Build history of the part. All positions in model axes, mm. A direction names the side the tool comes from. Round coordinates to 2 decimals unless told otherwise and drop trailing zeros. Write each loop counter-clockwise with the first axis right and the second up, starting at its lowest first coordinate (ties: lowest second). Pieces come first, ordered by that corner, then holes.
Autodesk Inventor part; units mm, degrees
ref_plane "YZ Plane" through (0, 0, 0) normal (1, 0, 0) x (0, 1, 0)
ref_plane "XZ Plane" through (0, 0, 0) normal (0, 1, 0) x (-1, 0, 0)
ref_plane "XY Plane" through (0, 0, 0) normal (0, 0, 1) x (1, 0, 0)
sketch "Sketch4" plane through (0, 0, 0) normal (0, 1, 0) x (-1, 0, 0)
  line L0 (0, 0) -> (12.35, 0)
  line L1 (12.35, 0) -> (12.35, -12.35)
  line L2 (12.35, -12.35) -> (8.925, -12.35)
  line L3 (8.925, -12.35) -> (8.925, -21.85)
  line L4 (8.925, -21.85) -> (1.425, -21.85)
  line L5 (1.425, -21.85) -> (1.425, -12.35)
  line L6 (1.425, -12.35) -> (0, -12.35)
  line L7 (0, -12.35) -> (0, 0)
  dimension "d17" = 12.35
  dimension "d18" = 12.35
  dimension "d19" = 7.5
  dimension "d20" = 1.425
  dimension "d21" = 9.5
extrude "Extrusion2" add sketch "Sketch4" along normal blind 8
sketch "Sketch5" plane through (0, 8, 0) normal (0, 1, 0) x (1, 0, 0)
  line L0 (-8.925, 14.35) -> (-6.425, 14.35)
  line L1 (-6.425, 14.35) -> (-6.425, 19.85)
  line L2 (-6.425, 19.85) -> (-8.925, 19.85)
  line L3 (-8.925, 19.85) -> (-8.925, 14.35)
  line L4 (-1.425, 21.85) -> (-8.925, 21.85)
  line L5 (-8.925, 21.85) -> (-8.925, 12.35)
  point P0 (0, 0)
  dimension "d24" = 5.5
  dimension "d25" = 2.5
  dimension "d26" = 2
extrude "Extrusion3" cut sketch "Sketch5" against normal through all
sketch "Sketch6" plane through (0, 8, 0) normal (0, 1, 0) x (1, 0, 0)
  circle A0 centre (-6.175, 6.175) radius 4.7625
  line L0 (-12.35, 0) -> (0, 0)
  line L1 (0, 0) -> (0, 12.35)
  dimension "d29" = 9.525
  dimension "d30" = 6.175
  dimension "d31" = 6.175
extrude "Extrusion4" cut sketch "Sketch6" against normal through all
sketch "Sketch7" plane through (0, 8, 0) normal (0, 1, 0) x (1, 0, 0)
  line L0 (-4.425, 8.85) -> (-3.425, 8.85)
  line L1 (-3.425, 8.85) -> (-3.425, 21.85)
  line L2 (-3.425, 21.85) -> (-4.425, 21.85)
  line L3 (-4.425, 21.85) -> (-4.425, 8.85)
  line L4 (-1.425, 21.85) -> (-8.925, 21.85)
  line L5 (-1.425, 12.35) -> (-1.425, 21.85)
  point P0 (0, 0)
  dimension "d34" = 1
  dimension "d35" = 13
  dimension "d36" = 2
extrude "Extrusion5" cut sketch "Sketch7" against normal through all
sketch "Sketch8" plane through (-1.425, 0, -12.35) normal (1, 0, 0) x (0, 0, -1)
  circle A0 centre (4.75, 4) radius 1.65
  line L0 (0, 0) -> (9.5, 0)
  line L1 (9.5, 0) -> (9.5, 8)
  point P0 (-12.35, 0)
  dimension "d39" = 3.3
  dimension "d40" = 4
  dimension "d41" = 4.75
extrude "Extrusion6" cut sketch "Sketch8" against normal through all
fillet "Fillet1" radius 2 4 edges at (-12.35, 4, -12.35) (-12.35, 4, 0) (0, 4, 0) (0, 4, -12.35)
sketch "Sketch9" plane through (-8.925, 0, -12.35) normal (-1, 0, 0) x (0, 0, 1)
  line L0 (-8.1, 4) -> (-6.425, 1.0988)
  line L1 (-6.425, 1.0988) -> (-3.075, 1.0988)
  line L2 (-3.075, 1.0988) -> (-1.4, 4)
  line L3 (-1.4, 4) -> (-3.075, 6.9012)
  line L4 (-3.075, 6.9012) -> (-6.425, 6.9012)
  line L5 (-6.425, 6.9012) -> (-8.1, 4)
  line L6 (-9.5, 8) -> (-7.5, 8)
  line L7 (-9.5, 0) -> (-9.5, 8)
  point P0 (12.35, 0)
  dimension "d46" = 3.35
  dimension "d47" = 3.35
  dimension "d48" = 3.35
  dimension "d49" = 3.35
  dimension "d50" = 3.35
  dimension "d51" = 120
  dimension "d52" = 120
  dimension "d53" = 4
  dimension "d55" = 6.425
extrude "Extrusion7" cut sketch "Sketch9" against normal blind 2.5
equation "\"d48\" = d46"
equation "\"d49\" = d47"
equation "\"d50\" = d47"
properties part number "COLLIER"
1) Pin check, flat tips, straight feed: pin 1 Ø3.5 at (y, z) = (3, -15.5) entering from -X (3 decimals); pin 2 Ø2.5 at (y, z) = (3, -16.5) entering from +X (3 decimals). Stop position of each tip, or through.
Results:
pin 1: stops at x = -8.925
pin 2: stops at x = -1.425
2) Slice it at A-A (z = -13.25). Write the cut outline in (x, y) (3 decimals).
Results:
outline: (-8.925, 0) - (-4.425, 0) - (-4.425, 8) - (-8.925, 8) - close; (-3.425, 0) - (-1.425, 0) - (-1.425, 8) - (-3.425, 8) - close
3) Which spindle directions (+Z, -Z, +X, -X, +Y, -Y) get a long thin tool onto all of the face, cutting with end or side? Do faces 5 (the flat face through (-8, 2, -14.35)), 6 (the flat face through (-1.425, 6, -17)), 7 (the flat face through (-7.693, 4.512, -14.046)), 8 (the flat face through (-10, 4, -12.35)). Say none if no direction does.
Results:
face 5: -X, +Y, -Y
face 6: -Z, +X, +Y, -Y
face 7: -X
face 8: -Z, -X, +Y, -Y
4) Slice it at D-D (z = -17.1). Write the cut outline in (x, y) (3 decimals).
Results:
outline: (-6.425, 0) - (-4.425, 0) - (-4.425, 2.35) - (-6.425, 2.35) - close; (-6.425, 5.65) - (-4.425, 5.65) - (-4.425, 8) - (-6.425, 8) - close; (-3.425, 0) - (-1.425, 0) - (-1.425, 2.35) - (-3.425, 2.35) - close; (-3.425, 5.65) - (-1.425, 5.65) - (-1.425, 8) - (-3.425, 8) - close
5) Mould opens along Z. For faces 1 (the flat face through (-4.425, 4, -15)), 2 (the cylindrical face through (-0.57, 3.94, -0.6)), 3 (the flat face through (-7.693, 3.488, -20.154)), 4 (the cylindrical face through (-11.78, 3.94, -11.75)) say: released by +Z, released by -Z, zero draft, split by the parting line, or undercut.
Results:
face 1: zero draft
face 2: released by +Z
face 3: undercut
face 4: released by -Z
6) Slice it at B-B (x = -9.75). Write the cut outline in (y, z).
Results:
outline: (0, -12.35) - (8, -12.35) - (8, -9.32) - (0, -9.32) - close; (0, -3.03) - (8, -3.03) - (8, 0) - (0, 0) - close
7) Wall check: L1, parallel to Y at x = -1.9, z = -17.1; L2, parallel to Z at x = -7, y = 7; L3, parallel to X at y = 3.5, z = -13 (3 decimals). Give the ranges that are in metal, low to high.
Results:
L1: y = 0 to 2.35, 5.65 to 8
L2: z = -21.85 to -19.85, -14.35 to -10.87, -1.48 to 0
L3: x = -8.925 to -4.425, -3.425 to -1.425
